from build123d import *
from build123d.topology import SkipClean

# Parameters (mm, degrees)
BOSS_EXTRUDE1_DEPTH = 12.5
CHAMFER1_SIZE       = 25
SKETCH3_W           = 35.35533906
SKETCH3_H           = 12.5
BOSS_EXTRUDE2_DEPTH = 20
SKETCH4_W           = 35.35533906
SKETCH4_H           = 12.5
BOSS_EXTRUDE3_DEPTH = 20
SKETCH5_W           = 35.35533906
SKETCH5_H           = 12.5
BOSS_EXTRUDE4_DEPTH = 20
SKETCH6_W           = 35.35533906
SKETCH6_H           = 12.5
BOSS_EXTRUDE5_DEPTH = 20
SHELL1_T            = -1
SKETCH7_R           = 1.5
CUT_EXTRUDE1_DEPTH  = 20
CIRPATTERN1_COUNT   = 4
SKETCH8_W           = 8
SKETCH8_H           = 75
BOSS_EXTRUDE6_DEPTH = 50
CUT_EXTRUDE2_REACH  = 167.514
SKETCH9_W           = 67
SKETCH9_H           = 42
FILLET2_START       = -38.388347648
FILLET2_DEPTH       = 8
FILLET2_START_2     = 30.388347648
FILLET2_2_DEPTH     = 8
FILLET2_START_3     = -42.5
FILLET2_3_DEPTH     = 85
FILLET2_START_4     = -44
FILLET2_4_OUTLINE_W = 1
FILLET2_4_OUTLINE_H = 67
FILLET2_4_DEPTH     = 88
FILLET3_R           = 5
CUT_EXTRUDE3_REACH  = 144.699
SKETCH10_W          = 33
SKETCH10_H          = 103
CUT_EXTRUDE4_START  = -12.5
SKETCH11_R          = 1.5
CUT_EXTRUDE4_DEPTH  = 12.5


with BuildPart() as part:
    # Sketch1 → Boss-Extrude1 (new body)
    with BuildSketch(Plane(origin=(0, 0, 0), x_dir=(1, 0, 0), z_dir=(0, 1, 0))):
        Polygon((88.388347648, 0), (0, 88.388347648), (-88.388347648, 0), (0, -88.388347648), align=None)
    extrude(amount=BOSS_EXTRUDE1_DEPTH)

    # Chamfer1
    chamfer1_edges = [part.edges().sort_by_distance(p)[0] for p in [
        (0, 6.25, 88.388347648),
        (-88.388347648, 6.25, 0),
        (0, 6.25, -88.388347648),
        (88.388347648, 6.25, 0),
    ]]
    chamfer(chamfer1_edges, length=CHAMFER1_SIZE)

    # Sketch3 → Boss-Extrude2 (add)
    with BuildSketch(Plane.XY.offset(70.710678119)):
        with Locations((0, 6.25)):
            Rectangle(SKETCH3_W, SKETCH3_H)
    extrude(amount=BOSS_EXTRUDE2_DEPTH)

    # Sketch4 → Boss-Extrude3 (add)
    with BuildSketch(Plane(origin=(70.710678119, 0, 0), x_dir=(0, 0, -1), z_dir=(1, 0, 0))):
        with Locations((0, 6.25)):
            Rectangle(SKETCH4_W, SKETCH4_H)
    extrude(amount=BOSS_EXTRUDE3_DEPTH)

    # Sketch5 → Boss-Extrude4 (add)
    with BuildSketch(Plane(origin=(0, 0, -70.710678119), x_dir=(-1, 0, 0), z_dir=(0, 0, -1))):
        with Locations((0, 6.25)):
            Rectangle(SKETCH5_W, SKETCH5_H)
    extrude(amount=BOSS_EXTRUDE4_DEPTH)

    # Sketch6 → Boss-Extrude5 (add)
    with BuildSketch(Plane.ZY.offset(70.710678119)):
        with Locations((0, 6.25)):
            Rectangle(SKETCH6_W, SKETCH6_H)
    extrude(amount=BOSS_EXTRUDE5_DEPTH)

    # Shell1
    shell1_openings = [part.faces().sort_by_distance(p)[0] for p in [
        (0, 6.25, 90.710678119),
        (90.710678119, 6.25, 0),
        (0, 6.25, -90.710678119),
        (-90.710678119, 6.25, 0),
    ]]
    offset(amount=SHELL1_T, openings=shell1_openings, kind=Kind.INTERSECTION)

    # Sketch7 → Cut-Extrude1 (cut)
    with BuildSketch(Plane(origin=(-70.710678119, 0, -17.67766953), x_dir=(1, 0, 0), z_dir=(0, 1, 0))):
        with Locations(Location((63.710678119, -88.388347648, 0), (0, 0, 270))):
            Circle(SKETCH7_R)
        with Locations(Location((77.710678119, -88.388347648, 0), (0, 0, 270))):
            Circle(SKETCH7_R)
    cut_extrude1 = extrude(amount=CUT_EXTRUDE1_DEPTH, mode=Mode.SUBTRACT)

    # CirPattern1: Cut-Extrude1 ×4 about axis
    cirpattern1_axis = Axis((0, 0, 0), (0, 1, 0))
    for i in range(1, CIRPATTERN1_COUNT):
        add(cut_extrude1.rotate(cirpattern1_axis, i * 360 / CIRPATTERN1_COUNT), mode=Mode.SUBTRACT)

    # Sketch8 → Boss-Extrude6 (add)
    with BuildSketch(Plane.XZ):
        with Locations((-34.388347648, 0)):
            Rectangle(SKETCH8_W, SKETCH8_H)
        with Locations((34.388347648, 0)):
            Rectangle(SKETCH8_W, SKETCH8_H)
    extrude(amount=BOSS_EXTRUDE6_DEPTH)

    # Cut-Extrude2: up to this face of the body (flat: up to its plane)
    cut_extrude2_end = Plane(part.part.faces().sort_by_distance((-38.388347648, -25, 0))[0])
    # Sketch9 → Cut-Extrude2 (cut, up to the picked face)
    with BuildSketch(Plane(origin=(38.388347648, 0, 0), x_dir=(0, 0, -1), z_dir=(1, 0, 0)), mode=Mode.PRIVATE) as cut_extrude2_sk1:
        with Locations((0, -25)):
            Rectangle(SKETCH9_W, SKETCH9_H)
    cut_extrude2_tool1 = split(extrude(cut_extrude2_sk1.sketch, amount=-CUT_EXTRUDE2_REACH, mode=Mode.PRIVATE), bisect_by=cut_extrude2_end, keep=Keep.BOTH, mode=Mode.PRIVATE)
    add(cut_extrude2_tool1.solids().sort_by(Axis((38.388348, -25, 0), (-1, 0, 0)))[0], mode=Mode.SUBTRACT)

    # Fillet2: read off the stored shape, not the designer's step
    # Fillet2 outline → Fillet2 (add)
    with BuildSketch(Plane.YZ.offset(FILLET2_START)):
        with BuildLine():
            Line((0, -42.5), (0, -37.5))
            Line((0, -37.5), (-5, -37.5))
            ThreePointArc((-5, -37.5), (-1.464466094, -38.964466094), (0, -42.5))
        make_face()
        with BuildLine():
            ThreePointArc((0, 42.5), (-1.464466094, 38.964466094), (-5, 37.5))
            Line((-5, 37.5), (0, 37.5))
            Line((0, 37.5), (0, 42.5))
        make_face()
    extrude(amount=FILLET2_DEPTH)

    # Fillet2 2 outline → Fillet2 2 (add)
    with BuildSketch(Plane.YZ.offset(FILLET2_START_2)):
        with BuildLine():
            Line((0, -42.5), (0, -37.5))
            Line((0, -37.5), (-5, -37.5))
            ThreePointArc((-5, -37.5), (-1.464466094, -38.964466094), (0, -42.5))
        make_face()
        with BuildLine():
            ThreePointArc((0, 42.5), (-1.464466094, 38.964466094), (-5, 37.5))
            Line((-5, 37.5), (0, 37.5))
            Line((0, 37.5), (0, 42.5))
        make_face()
    extrude(amount=FILLET2_2_DEPTH)

    # Fillet2 3 outline → Fillet2 3 (add)
    with BuildSketch(Plane.XY.offset(FILLET2_START_3)):
        with BuildLine():
            Line((-38.388347648, -5), (-38.388347648, 0))
            Line((-38.388347648, 0), (-43.388347648, 0))
            ThreePointArc((-43.388347648, 0), (-39.852813742, -1.464466094), (-38.388347648, -5))
        make_face()
        with BuildLine():
            ThreePointArc((-30.388347648, -5), (-28.923881554, -1.464466094), (-25.388347648, 0))
            Line((-25.388347648, 0), (-30.388347648, 0))
            Line((-30.388347648, 0), (-30.388347648, -5))
        make_face()
        with BuildLine():
            Line((43.388347648, 0), (38.388347648, 0))
            Line((38.388347648, 0), (38.388347648, -5))
            ThreePointArc((38.388347648, -5), (39.852813742, -1.464466094), (43.388347648, 0))
        make_face()
        with BuildLine():
            ThreePointArc((25.388347648, 0), (28.923881554, -1.464466094), (30.388347648, -5))
            Line((30.388347648, -5), (30.388347648, 0))
            Line((30.388347648, 0), (25.388347648, 0))
        make_face()
    extrude(amount=FILLET2_3_DEPTH)

    # Fillet2 4 outline → Fillet2 4 (cut)
    with SkipClean():  # the faces are left unmerged after this step: merging them gives an invalid solid
        with BuildSketch(Plane.YZ.offset(FILLET2_START_4)):
            with BuildLine():
                Line((-5, 42.5), (-5, 37.5))
                ThreePointArc((-5, 37.5), (-1.464466094, 38.964466094), (0, 42.5))
                Line((0, 42.5), (-5, 42.5))
            make_face()
            with BuildLine():
                Line((-5, -37.5), (-5, -42.5))
                Line((-5, -42.5), (0, -42.5))
                ThreePointArc((0, -42.5), (-1.464466094, -38.964466094), (-5, -37.5))
            make_face()
            with Locations((-4.5, 0)):
                Rectangle(FILLET2_4_OUTLINE_W, FILLET2_4_OUTLINE_H)
        extrude(amount=FILLET2_4_DEPTH, mode=Mode.SUBTRACT)
    add(part.part.scale(1), mode=Mode.REPLACE)  # the faces are merged on a copy

    # Fillet3
    fillet3_edges = [part.edges().sort_by_distance(p)[0] for p in [
        (-34.388347648, -50, -37.5),
        (-34.388347648, -50, 37.5),
        (34.388347648, -50, -37.5),
        (34.388347648, -50, 37.5),
    ]]
    fillet(fillet3_edges, radius=FILLET3_R)

    # Sketch10 → Cut-Extrude3 (cut, up to next)
    with BuildSketch(Plane(origin=(0, 12.5, 0), x_dir=(1, 0, 0), z_dir=(0, 1, 0)), mode=Mode.PRIVATE) as cut_extrude3_sk1:
        Rectangle(SKETCH10_W, SKETCH10_H)
    cut_extrude3_tool1 = extrude(cut_extrude3_sk1.sketch, amount=-CUT_EXTRUDE3_REACH, mode=Mode.PRIVATE) & part.part
    add(cut_extrude3_tool1.solids().sort_by_distance((0, 12.5, 0))[0], mode=Mode.SUBTRACT)

    # Sketch11 → Cut-Extrude4 (cut)
    with BuildSketch(Plane(origin=(0, 12.5, 0), x_dir=(1, 0, 0), z_dir=(0, 1, 0)).offset(CUT_EXTRUDE4_START)):
        with Locations(Location((0, -65.181873268, 0), (0, 0, 270))):
            Circle(SKETCH11_R)
        with Locations(Location((-65.181873268, 0, 0), (0, 0, 270))):
            Circle(SKETCH11_R)
        with Locations(Location((0, 65.181873268, 0), (0, 0, 270))):
            Circle(SKETCH11_R)
        with Locations(Location((65.181873268, 0, 0), (0, 0, 270))):
            Circle(SKETCH11_R)
    extrude(amount=CUT_EXTRUDE4_DEPTH, mode=Mode.SUBTRACT)


solid = part.part
Geometry check sheet. Reference: the model listing, model coordinates, mm. A direction names the side the tool comes from. Give positions to 0.01 mm unless a question says otherwise; leave off trailing zeros. Loops run counter-clockwise (first coordinate to the right, second up) from the corner with the lowest first, then second, coordinate; pieces in that order, holes last. Notation, with made-up numbers: (40.25, 14) -> (82.25, 14) arc R23 cw to (82.25, 51) -> close; hole circle Ø8 at (36.5, 20). An arc over 180 degrees is marked (long way). Answer in a Markdown table with one row per item. Add a question column.
1) Gauge pin test, flat ends, axial feed: P1, Ø6.5, axis at x = -36, y = -22.5, coming from the -Z side; P2, Ø4, axis at x = -70.71, z = -7, coming from the -Y side; P3, Ø4, axis at x = 33.5, y = -14.5, coming from the +Z side. Record the tip position at first contact, or that the pin passes through.
2) Cross-section at A-A on y = -16. Record the boundary of the cut face in (x, z).
3) Cross-section at C-C on y = 6.5. State how many separate pieces and enclosed holes the cut face has, and give its area (3 significant figures).
4) Cross-section at B-B on z = 54. Record the boundary of the cut face in (x, y), and give its area (3 significant figures).
5) Material ranges on probe 1 along X at (y, z) = (12, 0); probe 2 along Z at (x, y) = (0, 12.05); probe 3 along Y at (x, z) = (-32.5, 32), recorded low to high. Write a range as from..to.
6) Draft check along Y on faces 4 (the face through (-17.678, 6, 81)), 5 (the face through (-16.678, 6, 80)), 6 (the face through (34.262, -0.936, 39.587)). Enter one of: pulls with the +Y half, pulls with the -Y half, needs draft (parallel to the pull), parting line crosses it, or undercut.
7) Set-up check for faces 1 (the face through (-81, 6, -17.678)), 2 (the face through (34, -25, 37.5)), 3 (the face through (-34, -46, 0)): record each of +Z, -Z, +X, -X, +Y, -Y from which the full face is reachable in a straight line by a thin tool's end or side.
Outcome:
| question | item | result |
|---|---|---|
| 1 | P1 | stops at z = -37.5 |
| 1 | P2 | stops at y = 0 |
| 1 | P3 | stops at z = 37.5 |
| 2 | outline | (-38.39, -37.5) -> (-30.39, -37.5) -> (-30.39, -33.5) -> (-38.39, -33.5) -> close; (-38.39, 33.5) -> (-30.39, 33.5) -> (-30.39, 37.5) -> (-38.39, 37.5) -> close; (30.39, -37.5) -> (38.39, -37.5) -> (38.39, -33.5) -> (30.39, -33.5) -> close; (30.39, 33.5) -> (38.39, 33.5) -> (38.39, 37.5) -> (30.39, 37.5) -> close |
| 3 | separate pieces | 4 |
| 3 | enclosed holes | 0 |
| 3 | area | 463 mm^2 |
| 4 | outline | (-34.39, 0) -> (34.39, 0) -> (34.39, 12.5) -> (-34.39, 12.5) -> close; hole (-32.97, 1) -> (32.97, 1) -> (32.97, 11.5) -> (-32.97, 11.5) -> close |
| 4 | area | 167 mm^2 |
| 5 | probe 1 | x = -90.71..-66.68, -63.68..-16.5, 16.5..63.68, 66.68..90.71 |
| 5 | probe 2 | z = -90.71..-66.68, -63.68..-51.5, 51.5..63.68, 66.68..90.71 |
| 5 | probe 3 | y = -50..-46, -4..1, 11.5..12.5 |
| 6 | face 4 | needs draft |
| 6 | face 5 | undercut |
| 6 | face 6 | pulls with the -Y half |
| 7 | face 1 | -Z, -X, +Y, -Y |
| 7 | face 2 | +Z, +X, -X, -Y |
| 7 | face 3 | +X, -X |
